```python
from build123d import *

# Parameters (mm, degrees)
BOSS_EXTRUDE1_DEPTH = 130
BOSS_EXTRUDE2_DEPTH = 25
CHAMFER1_SIZE       = 2


with BuildPart() as part:
    # Sketch1 → Boss-Extrude1 (new body)
    with BuildSketch(Plane.XY):
        with BuildLine():
            Line((-8, 19), (8, 19))
            Line((8, 19), (8, 23.685438565))
            ThreePointArc((8, 23.685438565), (0, -25), (-8, 23.685438565))
            Line((-8, 23.685438565), (-8, 19))
        make_face()
    extrude(amount=BOSS_EXTRUDE1_DEPTH)

    # Sketch2 → Boss-Extrude2 (add)
    with BuildSketch(Plane(origin=(0, 0, 0), x_dir=(-1, 0, 0), z_dir=(0, 0, -1))):
        with BuildLine():
            Line((-8, 23.685438565), (-8, 19))
            Line((-8, 19), (8, 19))
            Line((8, 19), (8, 23.685438565))
            ThreePointArc((8, 23.685438565), (0, 25), (-8, 23.685438565))
        make_face()
    extrude(amount=-BOSS_EXTRUDE2_DEPTH)

    # Chamfer1
    chamfer1_edges = [part.edges().sort_by_distance(p)[0] for p in [
        (0, -25, 130),
        (8, -23.685438565, 0),
    ]]
    chamfer(chamfer1_edges, length=CHAMFER1_SIZE)


solid = part.part
```
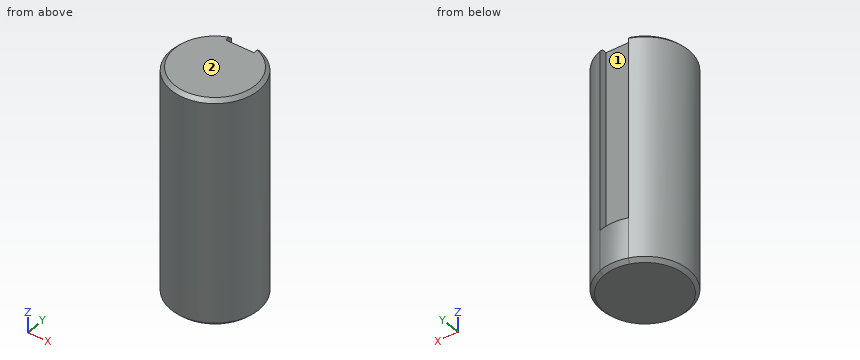
Check sheet for the modelled part. Datum: model origin and axes. Units: mm. Face numbers are marked on the shaded views. Round coordinates to 2 decimals unless told otherwise and drop trailing zeros. Order: outer loops, then holes, each group sorted by start corner. A loop starts at its lowest first (then second) coordinate and runs counter-clockwise, first axis right, second up.
1) Section check A-A (x = 0). Record the boundary of the cut face in (y, z), and give its area (3 significant figures).
2) Section check B-B (z = 58). Record the boundary of the cut face in (x, y).
3) Go/stop test with flat-tipped pins: pin 1 Ø4 at (x, z) = (-17, 79) entering from -Y; pin 2 Ø5 at (y, z) = (22, 73.5) entering from +X; pin 3 Ø3 at (x, z) = (-1, 88.5) entering from +Y. Record where each tip stops, or that it passes through.
4) Section check C-C (z = 16). Record the boundary of the cut face in (x, y), and give its area (3 significant figures).
5) Scan lines: line 1 (X direction, y = -1, z = 12); line 2 (X direction, y = 21, z = 84); line 3 (Z direction, x = -19, y = -13). Record each from-to range of solid material in increasing order.
6) Mould release check, pull along X, two halves, no side actions. Record for the marked faces 1 and 2: +X half, -X half, draft (parallel to the pull), parting line (faces both ways), or undercut.
Result:
1. outline: (-25, 2) - (-23, 0) - (23, 0) - (25, 2) - (25, 25) - (19, 25) - (19, 130) - (-23, 130) - (-25, 128) - close
1. area: 5,860 mm2
2. outline: (-8, 19) - (-8, 23.69) arc R25 ccw (long way) to (8, 23.69) - (8, 19) - close
3. pin 1: stops at y = -20
3. pin 2: stops at x = 15.64
3. pin 3: stops at y = 19
4. outline: circle Ø50 at (0, 0)
4. area: 1,960 mm2
5. line 1: x = -24.98 to 24.98
5. line 2: x = -13.56 to -8, 8 to 13.56
5. line 3: z = 0.02 to 129.98
6. face 1: undercut
6. face 2: draft
